```python
from build123d import *

# Parameters (mm, degrees)
SKETCH1_W           = 21
SKETCH1_H           = 2.5
BOSS_EXTRUDE1_DEPTH = 8.5
SKETCH2_W           = 2
SKETCH2_H           = 2
CUT_EXTRUDE1_DEPTH  = 5


with BuildPart() as part:
    # Sketch1 → Boss-Extrude1 (new body)
    with BuildSketch(Plane(origin=(0, 0, 0), x_dir=(1, 0, 0), z_dir=(0, 1, 0))):
        Rectangle(SKETCH1_W, SKETCH1_H)
    extrude(amount=BOSS_EXTRUDE1_DEPTH)

    # Sketch2 → Cut-Extrude1 (cut)
    with BuildSketch(Plane(origin=(0, 8.5, 0), x_dir=(1, 0, 0), z_dir=(0, 1, 0))):
        with Locations((-6.5, 0)):
            Rectangle(SKETCH2_W, SKETCH2_H)
        with Locations((-9, 0)):
            Rectangle(SKETCH2_W, SKETCH2_H)
        with Locations((-4, 0)):
            Rectangle(SKETCH2_W, SKETCH2_H)
        with Locations((-1.5, 0)):
            Rectangle(SKETCH2_W, SKETCH2_H)
        with Locations((1, 0)):
            Rectangle(SKETCH2_W, SKETCH2_H)
        with Locations((3.5, 0)):
            Rectangle(SKETCH2_W, SKETCH2_H)
        with Locations((6, 0)):
            Rectangle(SKETCH2_W, SKETCH2_H)
        with Locations((8.5, 0)):
            Rectangle(SKETCH2_W, SKETCH2_H)
    extrude(amount=-CUT_EXTRUDE1_DEPTH, mode=Mode.SUBTRACT)


solid = part.part
```
Here's how the part is built. I have some questions about the finished solid (model axes, mm). A direction names the side the tool comes from. Coordinates: 2 decimals unless noted, no trailing zeros. Order: outer loops, then holes, each group sorted by start corner. A loop starts at its lowest first (then second) coordinate and runs counter-clockwise, first axis right, second up. Notation, with made-up numbers: M 48,19.5 L 58,19.5 A21 cw 58,52.5 Z; hole C 1.25,59 d10. An arc over 180 degrees is marked long. Answer as a JSON object with one key per item and string values. Group by question number.
(1) Suppose I cut it at B-B, the plane y = 5.5. State how many separate pieces and enclosed holes the cut face has, then the cut area to 3 significant figures.
(2) I need wall thicknesses on probe 1 along Z at (x, y) = (5.25, 6); probe 2 along Y at (x, z) = (5.25, -0.35). Which ranges of each line are inside material? Lowest first, please.
(3) Suppose I cut it at A-A, the plane x = 0.25. Please give me the cut outline in (y, z), then the cut area to 4 significant figures.
(4) If we mould it in two halves opening along Z, with no side actions, what happens to faces 3 (the face through (10.5, 4, 0)), 4 (the face through (0, 4, -1.25)), 5 (the face through (-9, 3.5, 0))? For each: released by +Z, released by -Z, zero draft, split by the parting line, or undercut.
(5) Which directions (+Z, -Z, +X, -X, +Y, -Y) give clear straight access to the entire face, cutting with the end or side of a thin tool? Please do faces 1 (the face through (2.5, 6, 0)), 2 (the face through (0, 0, 0)).
Values found:
{
 "1": {"separate pieces": "1", "enclosed holes": "8", "area": "20.5 mm^2"},
 "2": {"probe 1": "z = -1.25 to -1, 1 to 1.25", "probe 2": "y = 0 to 3.5"},
 "3": {"outline": "M 0,-1.25 L 8.5,-1.25 L 8.5,-1 L 3.5,-1 L 3.5,1 L 8.5,1 L 8.5,1.25 L 0,1.25 Z", "area": "11.25 mm^2"},
 "4": {"face 3": "zero draft", "face 4": "released by -Z", "face 5": "undercut"},
 "5": {"face 1": "+Y", "face 2": "+Z, -Z, +X, -X, -Y"}
}
